Part model, mm, in its own coordinate system. A direction names the side the tool comes from. Coordinates: 2 decimals unless noted, no trailing zeros. Loops run counter-clockwise (first coordinate to the right, second up) from the corner with the lowest first, then second, coordinate; pieces in that order, holes last. Notation, with made-up numbers: M 81.25,-6.5 L 91.25,-6.5 A7 cw 91.25,3.5 Z; hole C 48,67.5 d5. An arc over 180 degrees is marked long. Use CSV: the item, a comma, the result in double quotes. Start each with the question number.
from build123d import *

# Parameters (mm, degrees)
SKETCH3_R               = 5
CUT_EXTRUDE1_DEPTH      = 23.2250001
CUT_EXTRUDE1_DEPTH_BACK = 443.2250001
SKETCH6_R               = 5
CUT_EXTRUDE2_DEPTH      = 803.225


with BuildPart() as part:
    # Sweep-Thin1: sweep along a path in Sketch1
    with BuildLine(Plane(origin=(0, 0, 0), x_dir=(1, 0, 0), z_dir=(0, 1, 0))) as sweep_thin1_path:
        Line((130, 0), (0, 0))
        Line((0, 0), (-610, 0))
        ThreePointArc((-610, 0), (-638.284271247, 11.715728753), (-650, 40))
        Line((-650, 40), (-650, 380))
        ThreePointArc((-650, 380), (-638.284271247, 408.284271247), (-610, 420))
        Line((-610, 420), (0, 420))
        Line((0, 420), (130, 420))
    # Sketch2 → Sweep-Thin1 (sweep)
    with BuildSketch(Plane(origin=(0, 0, 0), x_dir=(0, 0, -1), z_dir=(1, 0, 0))):
        with BuildLine():
            Line((14.05, 22.225), (-14.05, 22.225))
            ThreePointArc((-14.05, 22.225), (-19.830597936, 19.830597936), (-22.225, 14.05))
            Line((-22.225, 14.05), (-22.225, -14.05))
            ThreePointArc((-22.225, -14.05), (-19.830597936, -19.830597936), (-14.05, -22.225))
            Line((-14.05, -22.225), (14.05, -22.225))
            ThreePointArc((14.05, -22.225), (19.830597936, -19.830597936), (22.225, -14.05))
            Line((22.225, -14.05), (22.225, 14.05))
            ThreePointArc((22.225, 14.05), (19.830597936, 19.830597936), (14.05, 22.225))
        make_face()
        with BuildLine():
            Line((14.05, 19.05), (-14.05, 19.05))
            ThreePointArc((-14.05, 19.05), (-17.585533906, 17.585533906), (-19.05, 14.05))
            Line((-19.05, 14.05), (-19.05, -14.05))
            ThreePointArc((-19.05, -14.05), (-17.585533906, -17.585533906), (-14.05, -19.05))
            Line((-14.05, -19.05), (14.05, -19.05))
            ThreePointArc((14.05, -19.05), (17.585533906, -17.585533906), (19.05, -14.05))
            Line((19.05, -14.05), (19.05, 14.05))
            ThreePointArc((19.05, 14.05), (17.585533906, 17.585533906), (14.05, 19.05))
        make_face(mode=Mode.SUBTRACT)
    sweep(path=sweep_thin1_path.line)

    # Sketch3 → Cut-Extrude1 (cut, two sides)
    with BuildSketch(Plane.XY) as cut_extrude1_sk:
        with Locations((-50, 0)):
            Circle(SKETCH3_R)
    extrude(amount=CUT_EXTRUDE1_DEPTH, mode=Mode.SUBTRACT)
    extrude(cut_extrude1_sk.sketch, amount=-CUT_EXTRUDE1_DEPTH_BACK, mode=Mode.SUBTRACT)

    # Sketch6 → Cut-Extrude2 (cut, through all)
    with BuildSketch(Plane.ZY.offset(672.225)):
        with Locations((-210, 0)):
            Circle(SKETCH6_R)
    extrude(amount=-CUT_EXTRUDE2_DEPTH, mode=Mode.SUBTRACT)


solid = part.part
1. Two-plate mould, pull along X, no slides. Class faces 6 (the face through (-235, 0, -442.225)), 7 (the face through (-669.05, -6, -212)), 8 (the face through (-622.43, 0.197, -27.294)): pulls with the +X half, pulls with the -X half, needs draft (parallel to the pull), parting line crosses it, or undercut.
2. Wall check: probe 1 along Z at (x, y) = (-384.5, 3) (3 decimals); probe 2 along Y at (x, z) = (-260, -412.5) (3 decimals). Give the ranges that are in metal, low to high.
3. Slice it at B-B, the plane z = -195. List the corners of the cut face in (x, y) (3 decimals), and give its area (3 significant figures).
4. Tool access for faces 1 (the face through (-627.775, -6, -212)), 2 (the face through (130, -0.3, -439.4)), 3 (the face through (-654, 0, 4)), 4 (the face through (-652.211, 0.197, -421.293)), 5 (the face through (-235, 0, -400.95)): list every direction of +Z, -Z, +X, -X, +Y, -Y with a clear straight run to the whole face (end or side of a thin tool).
5. Slice it at A-A, the plane x = -301.5. State how many separate pieces and enclosed holes the cut face has, and give its area (3 significant figures).
6. Pin check, flat tips, straight feed: pin 1 (9 mm diameter, centred on y = 0, z = -210, fed in from +X); pin 2 (22.5 mm diameter, centred on y = -1.5, z = -221, fed in from +X) (3 decimals); pin 3 (6 mm diameter, centred on x = -410.5, y = 17.5, fed in from +Z). Stop position of each tip, or through.
Found:
1,face 6,"needs draft"
1,face 7,"undercut"
1,face 8,"pulls with the +X half"
2,probe 1,"-442.225 to -439.05, -400.95 to -397.775, -22.225 to -19.05, 19.05 to 22.225"
2,probe 2,"-22.225 to -19.05, 19.05 to 22.225"
3,outline,"M -672.225,-14.05 A8.175 ccw -664.05,-22.225 L -635.95,-22.225 A8.175 ccw -627.775,-14.05 L -627.775,14.05 A8.175 ccw -635.95,22.225 L -664.05,22.225 A8.175 ccw -672.225,14.05 Z; hole M -669.05,-14.05 A5 ccw -664.05,-19.05 L -635.95,-19.05 A5 ccw -630.95,-14.05 L -630.95,14.05 A5 ccw -635.95,19.05 L -664.05,19.05 A5 ccw -669.05,14.05 Z"
3,area,"488 mm^2"
4,face 1,"+X, +Y, -Y"
4,face 2,"+Z, -Z, +X, +Y, -Y"
4,face 3,"+Z, -X, +Y, -Y"
4,face 4,"none"
4,face 5,"+X"
5,separate pieces,"2"
5,enclosed holes,"2"
5,area,"977 mm^2"
6,pin 1,"through"
6,pin 2,"x = -627.775"
6,pin 3,"z = 22.21"
